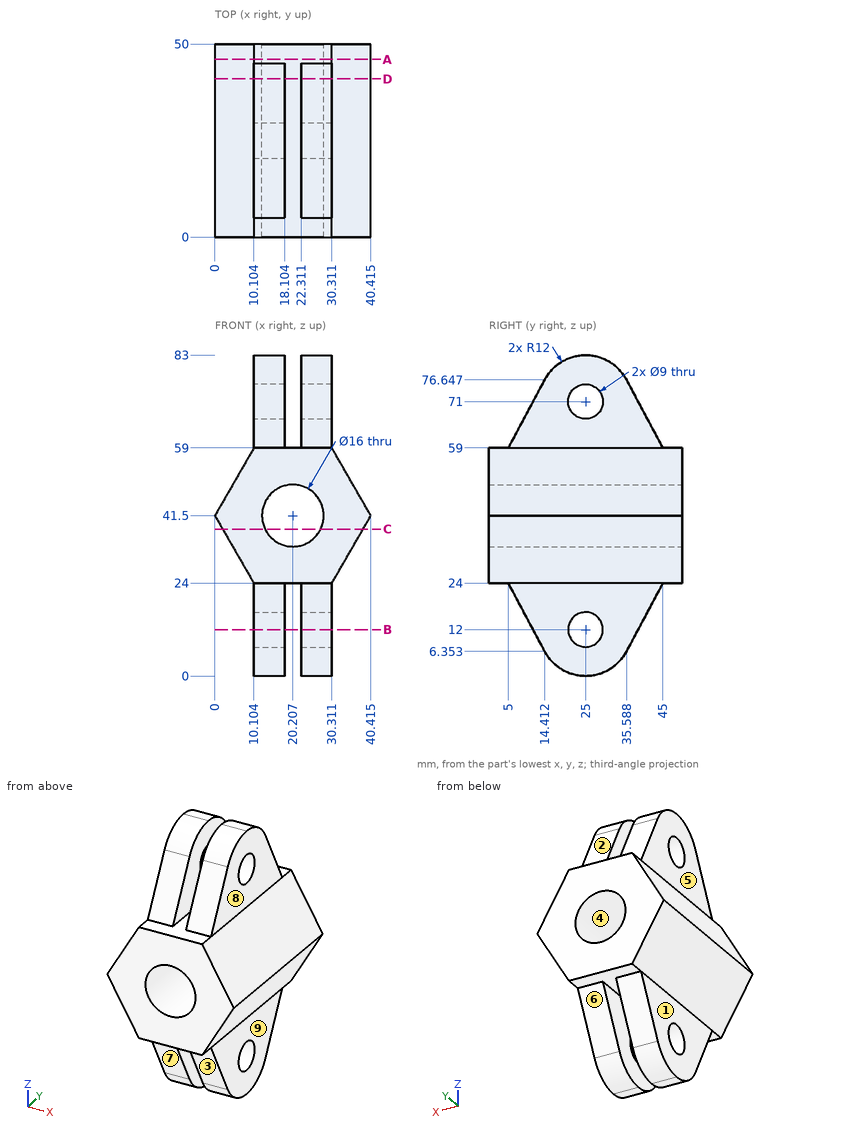
The drawing under review shows one solid part. Ordinate dimensions are in mm from its lowest x, y, z. A direction names the side the tool comes from. Coordinates: 2 decimals unless noted, no trailing zeros. Loops run counter-clockwise (first coordinate to the right, second up) from the corner with the lowest first, then second, coordinate; pieces in that order, holes last. Notation, with made-up numbers: M 86.25,65 L 121.25,65 A26 cw 121.25,101 Z; hole C -12,21 d6. An arc over 180 degrees is marked long. Use one line per item in the form item = value.
(1) For the marked faces 5, 6, 7, 8 and 9, list the 3-axis set-ups (+Z, -Z, +X, -X, +Y, -Y) from which the entire face can be reached by the end or side of a thin tool; tool diameter is ignored.
Return value:
face_5 = +Z, -X, +Y, -Y
face_6 = -Z, +X, -X, +Y
face_7 = -Z, +X, -X, -Y
face_8 = +Z, +X, +Y, -Y
face_9 = -Z, +X, +Y, -Y
(2) Consider section C-C (z = 38). Write out the cut boundary in (x, y), and give its area (3 significant figures).
Return value:
outline = M 2.02,0 L 13.01,0 L 13.01,50 L 2.02,50 Z; M 27.4,0 L 38.39,0 L 38.39,50 L 27.4,50 Z
area = 1,100 mm2
(3) Consider section B-B (z = 12). Write out the cut boundary in (x, y).
Return value:
outline = M 10.1,11.4 L 18.1,11.4 L 18.1,20.5 L 10.1,20.5 Z; M 10.1,29.5 L 18.1,29.5 L 18.1,38.6 L 10.1,38.6 Z; M 22.31,11.4 L 30.31,11.4 L 30.31,20.5 L 22.31,20.5 Z; M 22.31,29.5 L 30.31,29.5 L 30.31,38.6 L 22.31,38.6 Z
(4) Clearance check with flat-ended pins moving along their axes: P1, Ø19, axis at y = 17.5, z = 73.5, coming from the -X side; P2, Ø8, axis at y = 31, z = 61, coming from the +X side (1 decimal); P3, Ø2, axis at x = 15, y = 13.5, coming from the +Z side; P4, Ø7, axis at y = 25, z = 71, coming from the -X side. State where each tip first meets the part, or that it passes through.
Return value:
P1 = 10.1
P2 = 31.5
P3 = 76.81
P4 = through
(5) For line 1 along X through (y, z) = (25, 20); line 2 along Z through (x, y) = (14.75, 25); line 3 along X through (y, z) = (36.5, 46) (1 decimal), list the stretches that pass through material, from the lowest coordinate up. Write a range as from..to.
Return value:
line_1 = 10.1..18.1, 22.31..30.31
line_2 = 0..7.5, 16.5..35.65, 47.35..66.5, 75.5..83
line_3 = 2.6..13.6, 26.8..37.8
(6) Consider section A-A (y = 46). Write out the cut boundary in (x, z) (1 decimal), and give its area (3 significant figures).
Return value:
outline = M 0,41.5 L 10.1,24 L 30.3,24 L 40.4,41.5 L 30.3,59 L 10.1,59 Z; hole C 20.2,41.5 d16
area = 860 mm2
(7) Draft analysis for pull direction Z (two halves, no side actions). For the marked faces 1, 2, 3 and 4, state which applies: pulls with the +Z half, pulls with the -Z half, needs draft (parallel to the pull), parting line crosses it, or undercut.
Return value:
face_1 = needs draft
face_2 = pulls with the +Z half
face_3 = pulls with the -Z half
face_4 = undercut
(8) Consider section D-D (y = 41). Write out the cut boundary in (x, z) (1 decimal), and give its area (3 significant figures).
Return value:
outline = M 0,41.5 L 10.1,24 L 10.1,16.5 L 18.1,16.5 L 18.1,24 L 22.3,24 L 22.3,16.5 L 30.3,16.5 L 30.3,24 L 40.4,41.5 L 30.3,59 L 30.3,66.5 L 22.3,66.5 L 22.3,59 L 18.1,59 L 18.1,66.5 L 10.1,66.5 L 10.1,59 Z; hole C 20.2,41.5 d16
area = 1,100 mm2
